```python
from build123d import *

# Parameters (mm, degrees)
SKETCH1_W           = 60
SKETCH1_H           = 63
SKETCH1_R           = 4
SKETCH1_R_2         = 1.25
BOSS_EXTRUDE1_DEPTH = 1
FILLET1_R           = 3
SKETCH2_W           = 10
SKETCH2_H           = 5
BOSS_EXTRUDE2_DEPTH = 1
CHAMFER1_SIZE       = 1
CHAMFER2_SIZE       = 1


with BuildPart() as part:
    # Sketch1 → Boss-Extrude1 (new body)
    # profile 1 of 3: a face of its own
    with BuildSketch(Plane(origin=(0, 0, 0), x_dir=(1, 0, 0), z_dir=(0, 1, 0))):
        with Locations((30, 31.5)):
            Rectangle(SKETCH1_W, SKETCH1_H)
    # profile 2 of 3: a face of its own
    with BuildSketch(Plane(origin=(0, 0, 0), x_dir=(1, 0, 0), z_dir=(0, 1, 0))):
        with BuildLine():
            Line((26, 0), (26, -6))
            ThreePointArc((26, -6), (30, -2), (34, -6))
            Line((34, -6), (34, 0))
            Line((34, 0), (26, 0))
        make_face()
    # profile 3 of 3: a face of its own
    with BuildSketch(Plane(origin=(0, 0, 0), x_dir=(1, 0, 0), z_dir=(0, 1, 0))):
        with Locations((30, -6)):
            Circle(SKETCH1_R)
        with Locations(Location((30, -6, 0), (0, 0, 270))):
            Circle(SKETCH1_R_2, mode=Mode.SUBTRACT)
    extrude(amount=BOSS_EXTRUDE1_DEPTH)

    # Fillet1
    fillet1_edges = [part.edges().sort_by_distance(p)[0] for p in [
        (34, 0.5, 0),
        (26, 0.5, 0),
    ]]
    fillet(fillet1_edges, radius=FILLET1_R)

    # Sketch2 → Boss-Extrude2 (add)
    with BuildSketch(Plane(origin=(0, 0, 0), x_dir=(-1, 0, 0), z_dir=(0, -1, 0))):
        with Locations((-10, 63.5)):
            Rectangle(SKETCH2_W, SKETCH2_H)
        with Locations((-50, 63.5)):
            Rectangle(SKETCH2_W, SKETCH2_H)
    extrude(amount=BOSS_EXTRUDE2_DEPTH)

    # Chamfer1
    chamfer1_edges = [part.edges().sort_by_distance(p)[0] for p in [
        (50, 0, -61),
        (10, 0, -61),
    ]]
    chamfer(chamfer1_edges, length=CHAMFER1_SIZE - 0.0001)  # a hair under: the kernel refuses the full size

    # Chamfer2
    chamfer2_edges = [part.edges().sort_by_distance(p)[0] for p in [
        (30, 1, 4.75),
    ]]
    chamfer(chamfer2_edges, length=CHAMFER2_SIZE - 0.0001)  # a hair under: the kernel refuses the full size


solid = part.part
```
Work out the finished part from the listing and answer in its coordinate system (mm). A direction names the side the tool comes from. Coordinates: 2 decimals unless noted, no trailing zeros. Order: outer loops, then holes, each group sorted by start corner. A loop starts at its lowest first (then second) coordinate and runs counter-clockwise, first axis right, second up. Notation, with made-up numbers: (-38, -13.75) - (-7, -13.75) arc R21 cw to (-7, -0.75) - close; hole circle Ø10 at (50.5, 34). An arc over 180 degrees is marked (long way). Answer as a JSON object with one key per item and string values.
1. Find section D-D on x = 24. Determine the outline of the cut face in (y, z), plus the area to 3 significant figures.
Output values:
{"outline": "(0, -63) - (1, -63) - (1, 0.17) - (0, 0.17) - close", "area": "63.2 mm²"}
2. Consider line 1 (Y direction, x = 11, z = -33); line 2 (Z direction, x = 22, y = 0.9); line 3 (Z direction, x = 30.5, y = 0.4). Determine where each line is inside the solid, lowest interval first.
Output values:
{"line 1": "y = 0 to 1", "line 2": "z = -63 to 0", "line 3": "z = -63 to 4.43, 7.57 to 9.97"}
3. Find section B-B on y = 0.4. Determine the outline of the cut face in (x, z).
Output values:
{"outline": "(0, -63) - (60, -63) - (60, 0) - (37, 0) arc R3 cw to (34, 3) - (34, 6) arc R4 ccw to (26, 6) - (26, 3) arc R3 cw to (23, 0) - (0, 0) - close; hole circle Ø3.3 at (30, 6)"}
4. A tool of negligible diameter and unlimited length cuts with its end or side. For faces 1 (the face through (50, 0, -65)), 2 (the face through (30, 1, -27)), from which of +Z, -Z, +X, -X, +Y, -Y can it reach the whole face along a straight path? Write none if from no direction.
Output values:
{"face 1": "-Z, +X, -X, +Y", "face 2": "+Z, -Z, +X, -X, +Y"}
5. Find section C-C on z = -14. Determine the outline of the cut face in (x, y).
Output values:
{"outline": "(0, 0) - (60, 0) - (60, 1) - (0, 1) - close"}
6. Each of these flat-tipped pins is pushed along its axis until it touches: P1, Ø0.5, axis at y = -0.5, z = -63.5, coming from the +X side; P2, Ø4, axis at x = 41.5, z = -56.5, coming from the -Y side; P3, Ø2, axis at x = 30, z = 6, coming from the +Y side; P4, Ø0.8, axis at y = 0.5, z = 4.5, coming from the +X side. Where does it stop, or does it pass through?
Output values:
{"P1": "stops at x = 55", "P2": "stops at y = 0", "P3": "passes through", "P4": "stops at x = 34"}
